from build123d import *

# Parameters (mm, degrees)
SKETCH1_R           = 254
BOSS_EXTRUDE1_DEPTH = 12.7
SKETCH2_W           = 304.8
SKETCH2_H           = 304.8
CUT_EXTRUDE1_DEPTH  = 3.175
CUT_EXTRUDE2_DEPTH  = 3.175
SKETCH4_R           = 1.5
CUT_EXTRUDE3_DEPTH  = 360.434681131


with BuildPart() as part:
    # Sketch1 → Boss-Extrude1 (new body)
    with BuildSketch(Plane(origin=(0, 0, 0), x_dir=(1, 0, 0), z_dir=(0, 1, 0))):
        with Locations(Location((0, 0, 0), (0, 0, 270))):
            Circle(SKETCH1_R)
    extrude(amount=BOSS_EXTRUDE1_DEPTH)

    # Sketch2 → Cut-Extrude1 (cut)
    with BuildSketch(Plane(origin=(0, 12.7, 0), x_dir=(1, 0, 0), z_dir=(0, 1, 0))):
        Rectangle(SKETCH2_W, SKETCH2_H)
    extrude(amount=-CUT_EXTRUDE1_DEPTH, mode=Mode.SUBTRACT)

    # Sketch3 → Cut-Extrude2 (cut)
    with BuildSketch(Plane(origin=(0, 12.7, 0), x_dir=(1, 0, 0), z_dir=(0, 1, 0))):
        Polygon((94.954413465, 185.679071959), (98.836699141, 171.190184565), (113.325586535, 175.072470241), (109.443300859, 189.561357636), align=None)
        Polygon((218.886601718, 0), (208.28, 10.606601718), (197.673398282, 0), (208.28, -10.606601718), align=None)
        Polygon((109.443300859, -189.561357636), (113.325586535, -175.072470241), (98.836699141, -171.190184565), (94.954413465, -185.679071959), align=None)
        Polygon((-109.443300859, -189.561357636), (-94.954413465, -185.679071959), (-98.836699141, -171.190184565), (-113.325586535, -175.072470241), align=None)
        Polygon((-218.886601718, 0), (-208.28, -10.606601718), (-197.673398282, 0), (-208.28, 10.606601718), align=None)
        Polygon((-109.443300859, 189.561357636), (-113.325586535, 175.072470241), (-98.836699141, 171.190184565), (-94.954413465, 185.679071959), align=None)
    extrude(amount=-CUT_EXTRUDE2_DEPTH, mode=Mode.SUBTRACT)

    # Sketch4 → Cut-Extrude3 (cut, through all)
    with BuildSketch(Plane(origin=(0, 12.7, 0), x_dir=(1, 0, 0), z_dir=(0, 1, 0))):
        with Locations(Location((104.14, 180.3757711, 0), (0, 0, 270))):
            Circle(SKETCH4_R)
        with Locations(Location((208.28, 0, 0), (0, 0, 270))):
            Circle(SKETCH4_R)
        with Locations(Location((104.14, -180.3757711, 0), (0, 0, 270))):
            Circle(SKETCH4_R)
        with Locations(Location((-104.14, -180.3757711, 0), (0, 0, 270))):
            Circle(SKETCH4_R)
        with Locations(Location((-208.28, 0, 0), (0, 0, 270))):
            Circle(SKETCH4_R)
        with Locations(Location((-104.14, 180.3757711, 0), (0, 0, 270))):
            Circle(SKETCH4_R)
    extrude(amount=-CUT_EXTRUDE3_DEPTH, mode=Mode.SUBTRACT)


solid = part.part
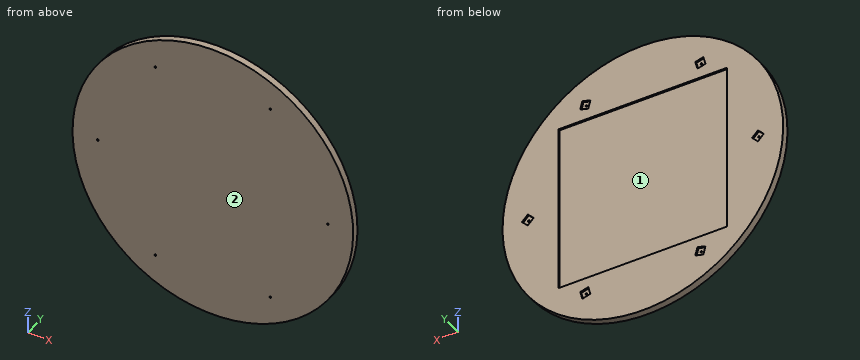
The model under review builds one solid part; all positions refer to its coordinate system, in mm. Face numbers are marked on the shaded views. Round coordinates to 2 decimals unless told otherwise and drop trailing zeros. Order: outer loops, then holes, each group sorted by start corner. A loop starts at its lowest first (then second) coordinate and runs counter-clockwise, first axis right, second up. Notation, with made-up numbers: (89.5, 24) - (131.5, 24) arc R12 ccw to (131.5, 29) - close; hole circle Ø9 at (-1.5, 33.5). An arc over 180 degrees is marked (long way). Use one line per item in the form item = value.
Q1. To check wall thickness, follow line 1 (X direction, y = 4.75, z = 0); line 2 (Z direction, x = 2.5, y = 1); line 3 (Z direction, x = -104.14, y = 4.5). State the ranges of each line that lie inside material, in increasing order.
Response values:
line_1 = -254 to -209.78, -206.78 to 206.78, 209.78 to 254
line_2 = -253.99 to 253.99
line_3 = -231.67 to -181.88, -178.88 to 178.88, 181.88 to 231.67
Q2. Clearance check with flat-ended pins moving along their axes: P1, Ø4, axis at x = 84.5, y = 3, coming from the -Z side; P2, Ø4, axis at x = -208.28, z = 0, coming from the +Y side (3 decimals); P3, Ø1, axis at y = 3, z = -29, coming from the +X side. State where each tip first meets the part, or that it passes through.
Response values:
P1 = -240.23
P2 = 9.525
P3 = 252.4
Q3. Add section B-B on x = 0. Give the boundary of the cut face in (y, z) (3 decimals), then the cut area to 3 significant figures.
Response values:
outline = (0, -254) - (12.7, -254) - (12.7, -152.4) - (9.525, -152.4) - (9.525, 152.4) - (12.7, 152.4) - (12.7, 254) - (0, 254) - close
area = 5,480 mm^2
Q4. Add section C-C on z = 61. Give the boundary of the cut face in (x, y) (3 decimals), then the cut area to 3 significant figures.
Response values:
outline = (-246.566, 0) - (246.566, 0) - (246.566, 12.7) - (152.4, 12.7) - (152.4, 9.525) - (-152.4, 9.525) - (-152.4, 12.7) - (-246.566, 12.7) - close
area = 5,300 mm^2
Q5. Add section D-D on x = -165.5. Give the boundary of the cut face in (y, z).
Response values:
outline = (0, -192.68) - (12.7, -192.68) - (12.7, 192.68) - (0, 192.68) - close
Q6. Mouldability with a two-part tool opening along X and no side actions: class the marked faces 1 and 2 as pulls with the +X half, pulls with the -X half, needs draft (parallel to the pull), parting line crosses it, or undercut.
Response values:
face_1 = undercut
face_2 = needs draft
Q7. Add section A-A on y = 2.75. Give the boundary of the cut face in (x, z), then the cut area to 3 significant figures.
Response values:
outline = circle Ø508 at (0, 0); hole circle Ø3 at (-208.28, 0); hole circle Ø3 at (-104.14, -180.38); hole circle Ø3 at (-104.14, 180.38); hole circle Ø3 at (104.14, -180.38); hole circle Ø3 at (104.14, 180.38); hole circle Ø3 at (208.28, 0)
area = 203,000 mm^2
